Read the model definition and answer for the solid it produces. Units are mm, in the model's axes. A direction names the side the tool comes from. Give positions to 0.01 mm unless a question says otherwise; leave off trailing zeros. Write each loop counter-clockwise with the first axis right and the second up, starting at its lowest first coordinate (ties: lowest second). Pieces come first, ordered by that corner, then holes. Notation, with made-up numbers: (-26, 61) -> (-20, 61) arc R20 cw to (-20, 72) -> close; hole circle Ø4 at (-26, 33). An arc over 180 degrees is marked (long way). Use a Markdown table: item, result.
Autodesk Inventor part; units mm, degrees
ref_plane "YZ Plane" through (0, 0, 0) normal (1, 0, 0) x (0, 1, 0)
ref_plane "XZ Plane" through (0, 0, 0) normal (0, 1, 0) x (-1, 0, 0)
ref_plane "XY Plane" through (0, 0, 0) normal (0, 0, 1) x (1, 0, 0)
sketch "Sketch1" plane through (0, 0, 0) normal (0, 0, 1) x (1, 0, 0)
  line L0 (-27.25, 33) -> (27.25, 33)
  line L1 (27.25, 33) -> (27.25, -33)
  line L2 (27.25, -33) -> (-27.25, -33)
  line L3 (-27.25, -33) -> (-27.25, 33)
  point P0 (0, 0)
  point P1 (0, 33)
  point P2 (-27.25, 0)
  dimension "d0" = 54.5
  dimension "d1" = 66
extrude "Extrusion1" add sketch "Sketch1" along normal blind 8
sketch "Sketch2" plane through (0, 0, 8) normal (0, 0, 1) x (1, 0, 0)
  line L0 (27.25, 33) -> (-27.25, 33)
  line L1 (-27.25, 33) -> (-27.25, -33)
  line L2 (-7.6866, 14.25) -> (7.6866, 14.25)
  line L3 (-12.41, -5.57) -> (-12.41, -14.27)
  line L4 (-13.515, -31) -> (-13.515, 8.4216)
  line L5 (13.515, 8.4216) -> (13.515, -31)
  line L6 (-27.25, -33) -> (27.25, -33)
  line L7 (-15.515, 16.25) -> (15.515, 16.25)
  line L8 (15.515, 16.25) -> (15.515, -33)
  line L9 (15.515, -33) -> (-15.515, -33)
  line L10 (-15.515, -33) -> (-15.515, 16.25)
  line L11 (-27.25, -33) -> (27.25, -33)
  point P0 (-27.25, 0)
  dimension "d29" = 2
  dimension "d30" = 2
  dimension "d32" = 2
extrude "Extrusion2" cut sketch "Sketch2" against normal through all
fillet "Fillet1" radius 1.5 2 edges at (-15.515, 16.25, 4) (15.515, 16.25, 4)
equation "\"d32\" = d30"
properties part number "0005-10-026 Suport DC in" material "Wood (Cherry)"
Item 1: Straight lines are drawn through the part: line 1 along X through (y, z) = (-7, 1.5) (3 decimals); line 2 along Y through (x, z) = (-3, 1.5). For each, find the intervals that lie inside material, in ascending order. Write a range as [from, to].
Return value:
| item | result |
|---|---|
| line 1 | [-27.25, -15.515], [15.515, 27.25] |
| line 2 | [16.25, 33] |
Item 2: This flat-tipped pin is pushed along its axis until it touches: P1, Ø2, axis at x = 2.5, z = 3, coming from the -Y side. Where does it stop, or does it pass through?
Return value:
| item | result |
|---|---|
| P1 | y = 16.25 |
Item 3: A tool of negligible diameter and unlimited length cuts with its end or side. For faces 1 (the face through (0, 33, 4)), 2 (the face through (15.064, 15.822, 3.944)), from which of +Z, -Z, +X, -X, +Y, -Y can it reach the whole face along a straight path? Write none if from no direction.
Return value:
| item | result |
|---|---|
| face 1 | +Z, -Z, +X, -X, +Y |
| face 2 | +Z, -Z, -Y |
Item 4: A cutting plane is placed at B-B (z = 2). Give the vertices of the cut face in (x, y) (3 decimals).
Return value:
| item | result |
|---|---|
| outline | (-27.25, -33) -> (-15.515, -33) -> (-15.515, 14.75) arc R1.5 cw to (-14.015, 16.25) -> (14.015, 16.25) arc R1.5 cw to (15.515, 14.75) -> (15.515, -33) -> (27.25, -33) -> (27.25, 33) -> (-27.25, 33) -> close |
Item 5: A cutting plane is placed at C-C (x = -6.5). Give the vertices of the cut face in (y, z), then the cut area to 3 significant figures.
Return value:
| item | result |
|---|---|
| outline | (16.25, 0) -> (33, 0) -> (33, 8) -> (16.25, 8) -> close |
| area | 134 mm^2 |
Item 6: A cutting plane is placed at A-A (y = 13.5). Give the vertices of the cut face in (x, z) (3 decimals).
Return value:
| item | result |
|---|---|
| outline | (-27.25, 0) -> (-15.515, 0) -> (-15.515, 8) -> (-27.25, 8) -> close; (15.515, 0) -> (27.25, 0) -> (27.25, 8) -> (15.515, 8) -> close |
